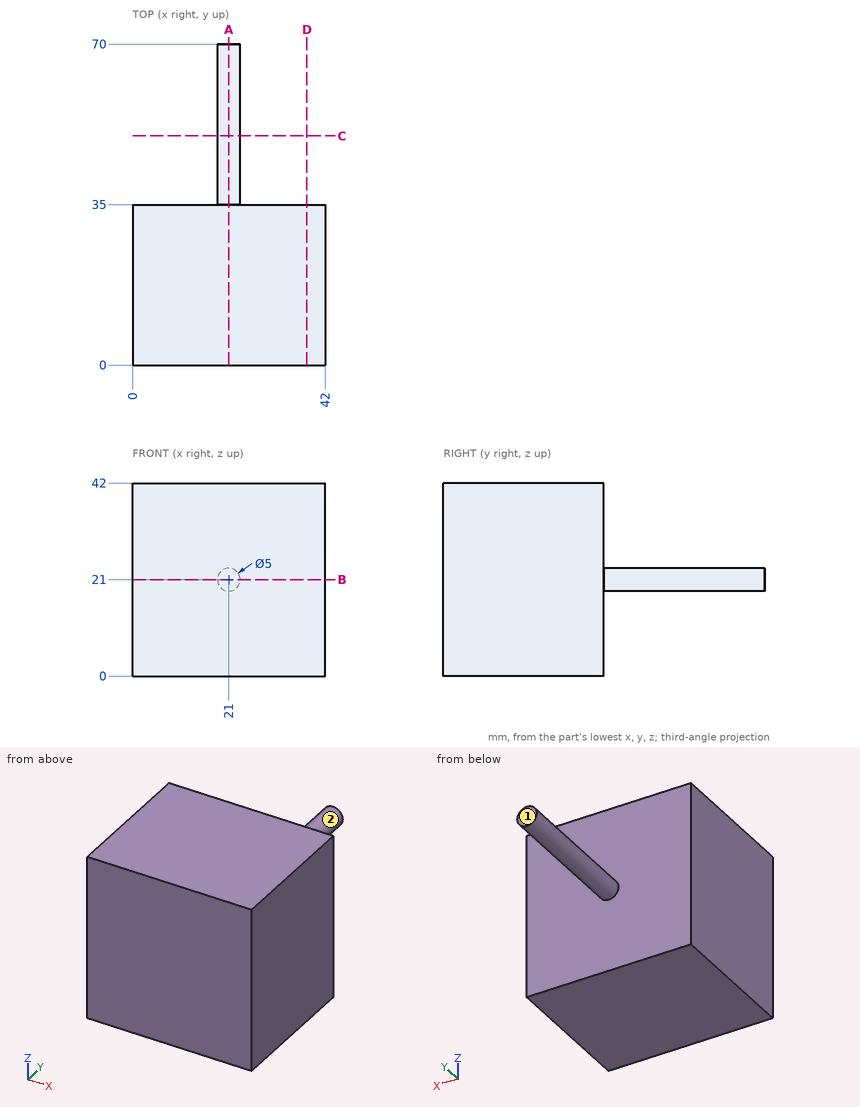
Here's the drawing with two shaded views (mm, measured from the low corner). I have some questions. A direction names the side the tool comes from. Give positions to 0.01 mm unless a question says otherwise; leave off trailing zeros. Loops run counter-clockwise (first coordinate to the right, second up) from the corner with the lowest first, then second, coordinate; pieces in that order, holes last. Notation, with made-up numbers: M 2,66.25 L 9,66.25 A27 ccw 9,87.25 Z; hole C 61.5,21.25 d2. An arc over 180 degrees is marked long. Answer in a Markdown table with one row per item.
1. Which directions (+Z, -Z, +X, -X, +Y, -Y) give clear straight access to the entire face, cutting with the end or side of a thin tool? Please do the marked faces 1 and 2.
Taken from the geometry:
| item | result |
|---|---|
| face 1 | +Z, -Z, +X, -X, +Y |
| face 2 | +Y |
2. Suppose I cut it at D-D on x = 38. Write out the boundary of the cut face in (y, z).
Taken from the geometry:
| item | result |
|---|---|
| outline | M 0,0 L 35,0 L 35,42 L 0,42 Z |
3. If I drill on line 1 along Y through (x, z) = (2.5, 38); line 2 along X through (y, z) = (36.5, 20), over which ranges is the centre line in solid material (lowest first)?
Taken from the geometry:
| item | result |
|---|---|
| line 1 | y = 0 to 35 |
| line 2 | x = 18.71 to 23.29 |
4. Suppose I cut it at B-B on z = 21. Write out the boundary of the cut face in (x, y).
Taken from the geometry:
| item | result |
|---|---|
| outline | M 0,0 L 42,0 L 42,35 L 23.5,35 L 23.5,70 L 18.5,70 L 18.5,35 L 0,35 Z |
5. Suppose I cut it at C-C on y = 50. Write out the boundary of the cut face in (x, z), plus the area to 3 significant figures.
Taken from the geometry:
| item | result |
|---|---|
| outline | C 21,21 d5 |
| area | 19.6 mm² |
6. For pin 1 Ø1 at (x, z) = (32, 28.5) entering from +Y, with a flat end and sliding along its axis, tell me the tip position at first contact or that it passes through.
Taken from the geometry:
| item | result |
|---|---|
| pin 1 | stops at y = 35 |
7. Suppose I cut it at A-A on x = 21. Write out the boundary of the cut face in (y, z), plus the area to 4 significant figures.
Taken from the geometry:
| item | result |
|---|---|
| outline | M 0,0 L 35,0 L 35,18.5 L 70,18.5 L 70,23.5 L 35,23.5 L 35,42 L 0,42 Z |
| area | 1,645 mm² |
